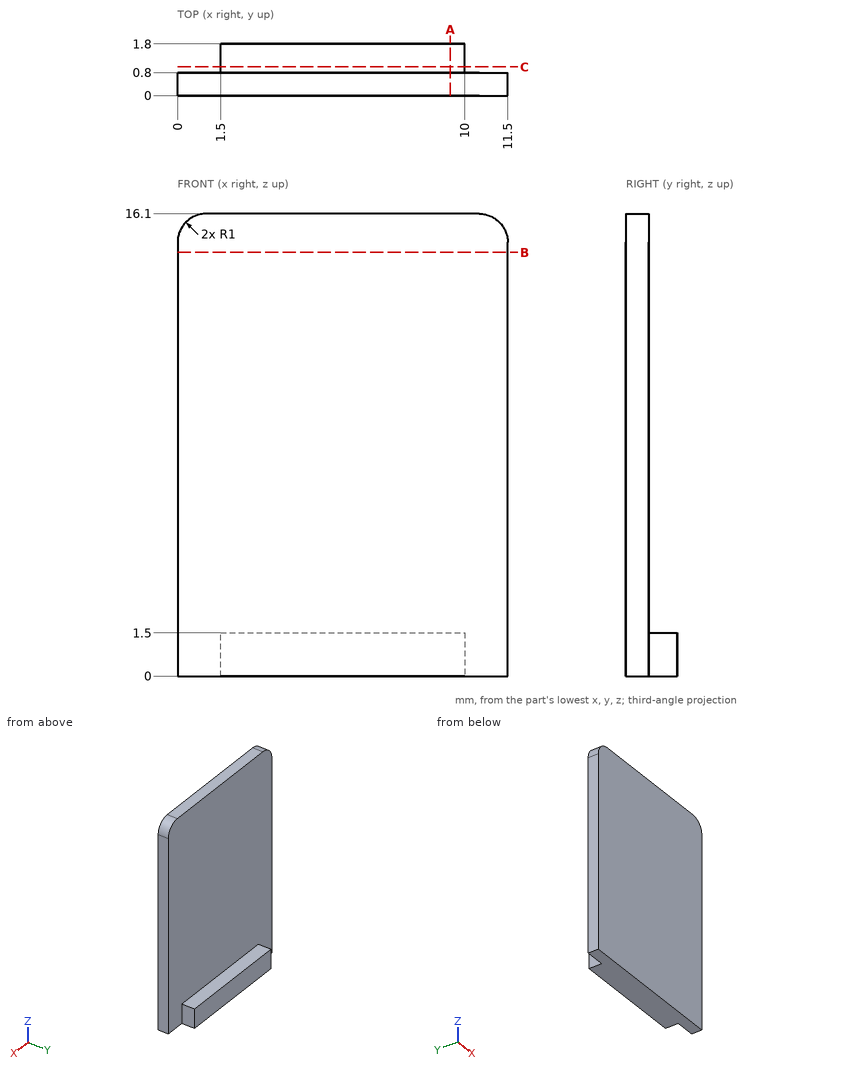
Here's the drawing with two shaded views (mm, measured from the low corner). I have some questions. Round coordinates to 2 decimals unless told otherwise and drop trailing zeros. Loops run counter-clockwise (first coordinate to the right, second up) from the corner with the lowest first, then second, coordinate; pieces in that order, holes last. Notation, with made-up numbers: M 37,26.25 L 85,26.25 A15 cw 85,54.25 Z; hole C 62,77 d11. An arc over 180 degrees is marked long. Answer as a JSON object with one key per item and string values. Group by question number.
Q1. Imagine slicing it at B-B, the plane z = 14.75. Please give me the cut outline in (x, y).
Q2. Imagine slicing it at C-C, the plane y = 1. Please give me the cut outline in (x, z).
Q3. Please list where these lines run through material, in increasing order: L1, parallel to Y at x = 5, z = 9; L2, parallel to Z at x = 6, y = 1.3.
Q4. Imagine slicing it at A-A, the plane x = 9.5. Please give me the cut outline in (y, z).
Q5. Will these pins go through, and if not, where does the flat tip stop? pin 1 (3.5 mm diameter, centred on x = 8.5, z = 9, fed in from +Y); pin 2 (1 mm diameter, centred on x = 2, y = 1.5, fed in from +Z); pin 3 (0.8 mm diameter, centred on x = 6, y = 1, fed in from +Z).
Findings:
{
 "1": {"outline": "M 0,0 L 11.5,0 L 11.5,0.8 L 0,0.8 Z"},
 "2": {"outline": "M 1.5,0 L 10,0 L 10,1.5 L 1.5,1.5 Z"},
 "3": {"L1": "y = 0 to 0.8", "L2": "z = 0 to 1.5"},
 "4": {"outline": "M 0,0 L 1.8,0 L 1.8,1.5 L 0.8,1.5 L 0.8,16.1 L 0,16.1 Z"},
 "5": {"pin 1": "stops at y = 0.8", "pin 2": "stops at z = 1.5", "pin 3": "stops at z = 16.1"}
}
